For this review, take the finished solid that the model builds, in its own axes (mm). Round coordinates to 2 decimals unless told otherwise and drop trailing zeros. Write each loop counter-clockwise with the first axis right and the second up, starting at its lowest first coordinate (ties: lowest second). Pieces come first, ordered by that corner, then holes. Notation, with made-up numbers: (23.5, 10.25) -> (51.5, 10.25) arc R30 ccw to (51.5, 37.25) -> close; hole circle Ø5 at (-1, 72). An arc over 180 degrees is marked (long way). Answer in a Markdown table with one row per item.
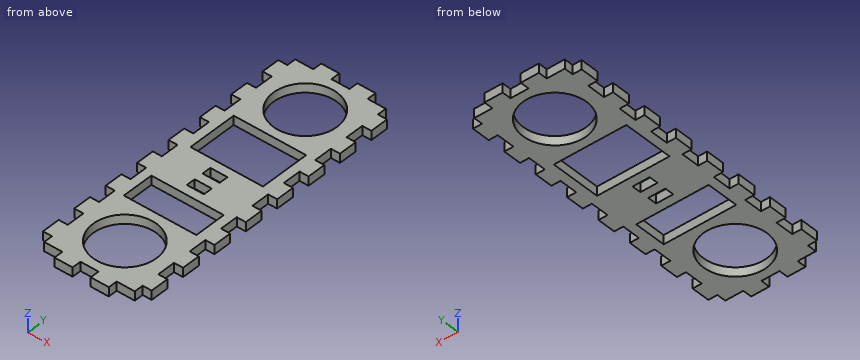
from build123d import *

# Parameters (mm, degrees)
F0_W     = 38.1
F0_H     = 107.95
F0_R     = 11.1125
F1_DEPTH = 3.175
F2_W     = 3.175
F2_H     = 6.35
F2_H_2   = 3.175
F2_W_2   = 25.4
F2_H_3   = 17.4625
F2_W_3   = 6
F2_H_4   = 11.1125
F3_DEPTH = 3.175
F4_W     = 6.35
F4_H     = 3.175
F5_DEPTH = 3.175


with BuildPart() as f1:
    # F0 (on Top) → F1 (new body)
    with BuildSketch(Plane.XY):
        with Locations((19.05, -53.975)):
            Rectangle(F0_W, F0_H)
        with Locations((19.05, -90.4875)):
            Circle(F0_R, mode=Mode.SUBTRACT)
        with Locations((19.05, -17.4625)):
            Circle(F0_R, mode=Mode.SUBTRACT)
    extrude(amount=F1_DEPTH)

    # F2 (on face) → F3 (cut, through all)
    with BuildSketch(Plane.XY.offset(3.175)):
        with Locations((36.5125, -3.175)):
            Rectangle(F2_W, F2_H)
        with Locations((1.5875, -3.175)):
            Rectangle(F2_W, F2_H)
        with Locations((1.5875, -15.875)):
            Rectangle(F2_W, F2_H)
        with Locations((36.5125, -15.875)):
            Rectangle(F2_W, F2_H)
        with Locations((36.5125, -28.575)):
            Rectangle(F2_W, F2_H)
        with Locations((36.5125, -41.275)):
            Rectangle(F2_W, F2_H)
        Polygon((22.05, -55.5625), (22.05, -53.975), (22.05, -52.3875), (16.05, -52.3875), (16.05, -55.5625), align=None)
        with Locations((36.5125, -52.3875)):
            Rectangle(F2_W, F2_H_2)
        with Locations((36.5125, -55.5625)):
            Rectangle(F2_W, F2_H_2)
        with Locations((36.5125, -66.675)):
            Rectangle(F2_W, F2_H)
        with Locations((36.5125, -79.375)):
            Rectangle(F2_W, F2_H)
        with Locations((36.5125, -92.075)):
            Rectangle(F2_W, F2_H)
        with Locations((36.5125, -104.775)):
            Rectangle(F2_W, F2_H)
        with Locations((36.5125, -117.475)):
            Rectangle(F2_W, F2_H)
        with Locations((36.5125, -130.175)):
            Rectangle(F2_W, F2_H)
        with Locations((1.5875, -28.575)):
            Rectangle(F2_W, F2_H)
        with Locations((1.5875, -41.275)):
            Rectangle(F2_W, F2_H)
        with Locations((1.5875, -53.975)):
            Rectangle(F2_W, F2_H)
        with Locations((1.5875, -66.675)):
            Rectangle(F2_W, F2_H)
        with Locations((1.5875, -79.375)):
            Rectangle(F2_W, F2_H)
        with Locations((1.5875, -92.075)):
            Rectangle(F2_W, F2_H)
        with Locations((1.5875, -104.775)):
            Rectangle(F2_W, F2_H)
        with Locations((1.5875, -117.475)):
            Rectangle(F2_W, F2_H)
        with Locations((1.5875, -130.175)):
            Rectangle(F2_W, F2_H)
        with Locations((19.05, -40.48125)):
            Rectangle(F2_W_2, F2_H_3)
        with Locations((19.05, -60.325)):
            Rectangle(F2_W_3, F2_H_2)
        with Locations((19.05, -70.64375)):
            Rectangle(F2_W_2, F2_H_4)
    extrude(amount=-F3_DEPTH, mode=Mode.SUBTRACT)

    # F4 (on face) → F5 (cut, through all)
    with BuildSketch(Plane.XY.offset(3.175)):
        with Locations((19.05, -1.5875)):
            Rectangle(F4_W, F4_H)
        with Locations((31.75, -1.5875)):
            Rectangle(F4_W, F4_H)
        with Locations((6.35, -1.5875)):
            Rectangle(F4_W, F4_H)
        with Locations((31.75, -106.3625)):
            Rectangle(F4_W, F4_H)
        with Locations((6.35, -106.3625)):
            Rectangle(F4_W, F4_H)
        with Locations((19.05, -106.3625)):
            Rectangle(F4_W, F4_H)
    extrude(amount=-F5_DEPTH, mode=Mode.SUBTRACT)


solid = f1.part
1) Consider section B-B on y = -87. State the section outline as (x, z) points (3 decimals), then the cut area to 3 significant figures.
Solved:
| item | result |
|---|---|
| outline | (0, 0) -> (8.499, 0) -> (8.499, 3.175) -> (0, 3.175) -> close; (29.601, 0) -> (38.1, 0) -> (38.1, 3.175) -> (29.601, 3.175) -> close |
| area | 54.0 mm² |
2) For line 1 (X direction, y = -33, z = 0.1); line 2 (Y direction, x = 25, z = 1.3); line 3 (X direction, y = -65, z = 0.55) (3 decimals), list the stretches that pass through material, from the lowest coordinate up. Write a range as [from, to].
Solved:
| item | result |
|---|---|
| line 1 | [0, 6.35], [31.75, 38.1] |
| line 2 | [-107.95, -99.87], [-81.1, -76.2], [-65.09, -49.21], [-31.75, -26.85], [-8.08, 0] |
| line 3 | [3.175, 34.925] |
3) Clearance check with flat-ended pins moving along their axes: pin 1 Ø1 at (y, z) = (-2, 2) entering from +X (3 decimals); pin 2 Ø1 at (y, z) = (-91.5, 2.5) entering from -X (3 decimals); pin 3 Ø1.6 at (y, z) = (-29.5, 1) entering from +X (3 decimals); pin 4 Ø2 at (x, y) = (25, -11) entering from +Z. State where each tip first meets the part, or that it passes through.
Solved:
| item | result |
|---|---|
| pin 1 | x = 28.575 |
| pin 2 | x = 3.175 |
| pin 3 | x = 34.925 |
| pin 4 | through |
4) Consider section A-A on x = 19.05. State how many separate pieces and enclosed holes the cut face has, then the cut area to 3 significant figures.
Solved:
| item | result |
|---|---|
| separate pieces | 7 |
| enclosed holes | 0 |
| area | 70.6 mm² |
5) Consider section D-D on x = 33. State the section outline as (y, z) points (3 decimals), then the cut area to 3 significant figures.
Solved:
| item | result |
|---|---|
| outline | (-104.775, 0) -> (-3.175, 0) -> (-3.175, 3.175) -> (-104.775, 3.175) -> close |
| area | 323 mm² |
